from build123d import *

# Parameters (mm, degrees)
BOSS_EXTRUDE1_DEPTH = 12.7


with BuildPart() as part:
    # Sketch2 → Boss-Extrude1 (new body)
    with BuildSketch(Plane(origin=(0, 0, 0), x_dir=(1, 0, 0), z_dir=(0, 1, 0))):
        Polygon((0, 44.45), (-31.75, 25.4), (-31.75, -25.4), (0, -44.45), (76.2, -44.45), (107.95, -25.4), (107.95, 25.4), (76.2, 44.45), align=None)
        with BuildLine():
            Line((0, 12.7), (76.2, 12.7))
            ThreePointArc((76.2, 12.7), (88.9, 0), (76.2, -12.7))
            Line((76.2, -12.7), (0, -12.7))
            ThreePointArc((0, -12.7), (-12.7, 0), (0, 12.7))
        make_face(mode=Mode.SUBTRACT)
    extrude(amount=BOSS_EXTRUDE1_DEPTH)


solid = part.part
Design review of the part built by this model. Coordinates are the model's own, in mm. A direction names the side the tool comes from. Give positions to 0.01 mm unless a question says otherwise; leave off trailing zeros. Loops run counter-clockwise (first coordinate to the right, second up) from the corner with the lowest first, then second, coordinate; pieces in that order, holes last. Notation, with made-up numbers: M -4,7 L 40,7 A13 ccw 40,14 Z; hole C 86.25,37 d1. An arc over 180 degrees is marked long. Answer as a JSON object with one key per item and string values.
Item 1: We need section C-C (y = 7.25). State the section outline as (x, z) points.
Output values:
{"outline": "M -31.75,-25.4 L 0,-44.45 L 76.2,-44.45 L 107.95,-25.4 L 107.95,25.4 L 76.2,44.45 L 0,44.45 L -31.75,25.4 Z; hole M 0,-12.7 L 76.2,-12.7 A12.7 ccw 76.2,12.7 L 0,12.7 A12.7 ccw Z"}
Item 2: For P1, Ø1, axis at x = -4.5, z = 31, coming from the -Y side, flat-tipped, find the tip position at first contact; note if it passes through.
Output values:
{"P1": "stops at y = 0"}
Item 3: Machinability: for faces 1 (the face through (-16.1, 6.26, 34.79)), 2 (the face through (-12.697, 6.261, 0.279)), which of the approach directions +Z, -Z, +X, -X, +Y, -Y give a long, thin tool a straight path to every point of the face, cutting with its end or side? Answer none if there is none.
Output values:
{"face 1": "+Z, -X, +Y, -Y", "face 2": "+Y, -Y"}
Item 4: We need section B-B (z = 0). State the section outline as (x, y) points.
Output values:
{"outline": "M -31.75,0 L -12.7,0 L -12.7,12.7 L -31.75,12.7 Z; M 88.9,0 L 107.95,0 L 107.95,12.7 L 88.9,12.7 Z"}
Item 5: We need section D-D (z = -34). State the section outline as (x, y) points.
Output values:
{"outline": "M -17.42,0 L 93.62,0 L 93.62,12.7 L -17.42,12.7 Z"}
Item 6: We need section A-A (x = 40.5). State the section outline as (y, z) points, and give its area (3 significant figures).
Output values:
{"outline": "M 0,-44.45 L 12.7,-44.45 L 12.7,-12.7 L 0,-12.7 Z; M 0,12.7 L 12.7,12.7 L 12.7,44.45 L 0,44.45 Z", "area": "806 mm2"}
Item 7: Mouldability with a two-part tool opening along X and no side actions: class faces 3 (the face through (-15.65, 6.26, -35.06)), 4 (the face through (88.897, 6.261, -0.279)), 5 (the face through (107.95, 6, 0)) as pulls with the +X half, pulls with the -X half, needs draft (parallel to the pull), parting line crosses it, or undercut.
Output values:
{"face 3": "pulls with the -X half", "face 4": "undercut", "face 5": "pulls with the +X half"}
Item 8: Wall thickness on line 1 along Z through (x, y) = (24.5, 5.75); line 2 along X through (y, z) = (0.5, -0.5); line 3 along X through (y, z) = (9.75, -2): over which ranges is each line inside the solid? List them lowest first.
Output values:
{"line 1": "z = -44.45 to -12.7, 12.7 to 44.45", "line 2": "x = -31.75 to -12.69, 88.89 to 107.95", "line 3": "x = -31.75 to -12.54, 88.74 to 107.95"}
